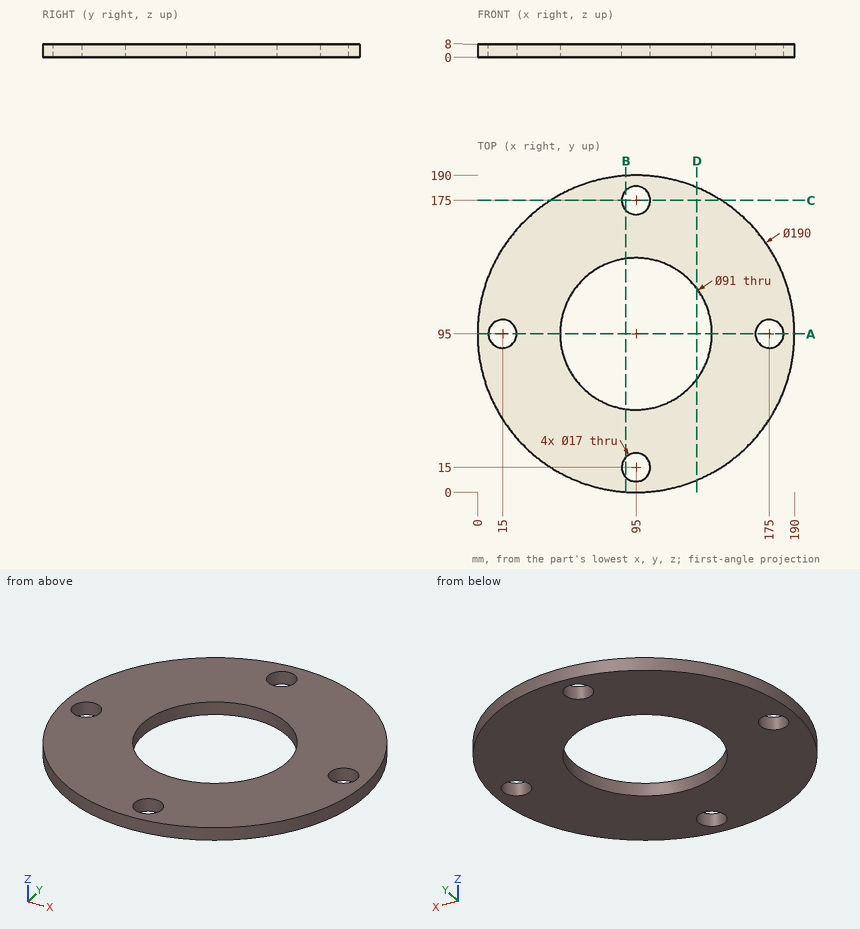
The figure shows three views and two pictorial views of one solid part (mm, origin at its lowest corner). Answer the questions. Give positions to 0.01 mm unless a question says otherwise; leave off trailing zeros. Write each loop counter-clockwise with the first axis right and the second up, starting at its lowest first coordinate (ties: lowest second). Pieces come first, ordered by that corner, then holes.
Q1. Given pin 1 (1 mm diameter, centred on y = 144.5, z = 5.5, fed in from +X); pin 2 (3 mm diameter, centred on x = 62.5, z = 5.5, fed in from +Y); pin 3 (15.5 mm diameter, centred on x = 15, y = 95, fed in from +Z); pin 4 (1.5 mm diameter, centred on x = 127, z = 3, fed in from +Y), each flat-ended and moving along its own axis, determine where each tip first touches the part or whether it passes through.
Answer:
pin 1: stops at x = 176.39
pin 2: stops at y = 184.8
pin 3: passes through
pin 4: stops at y = 184.71
Q2. The part is cut by section A-A on y = 95. Give the vertices of the cut face in (x, z).
Answer:
outline: (0, 0) - (6.5, 0) - (6.5, 8) - (0, 8) - close; (23.5, 0) - (49.5, 0) - (49.5, 8) - (23.5, 8) - close; (140.5, 0) - (166.5, 0) - (166.5, 8) - (140.5, 8) - close; (183.5, 0) - (190, 0) - (190, 8) - (183.5, 8) - close
Q3. The part is cut by section B-B on x = 89. Give the vertices of the cut face in (y, z), and give its area (3 significant figures).
Answer:
outline: (0.19, 0) - (8.98, 0) - (8.98, 8) - (0.19, 8) - close; (21.02, 0) - (49.9, 0) - (49.9, 8) - (21.02, 8) - close; (140.1, 0) - (168.98, 0) - (168.98, 8) - (140.1, 8) - close; (181.02, 0) - (189.81, 0) - (189.81, 8) - (181.02, 8) - close
area: 603 mm2
Q4. Straight lines are drawn through the part: L1, parallel to Y at x = 95.5, z = 7.5; L2, parallel to X at y = 17, z = 3; L3, parallel to Y at x = 73.5, z = 6.25. For each, find the intervals that lie inside material, in ascending order.
Answer:
L1: y = 0 to 6.51, 23.49 to 49.5, 140.5 to 166.51, 183.49 to 190
L2: x = 40.77 to 86.74, 103.26 to 149.23
L3: y = 2.46 to 54.9, 135.1 to 187.54
Q5. The part is cut by section C-C on y = 175. Give the vertices of the cut face in (x, z), and give its area (3 significant figures).
Answer:
outline: (43.77, 0) - (86.5, 0) - (86.5, 8) - (43.77, 8) - close; (103.5, 0) - (146.23, 0) - (146.23, 8) - (103.5, 8) - close
area: 684 mm2
Q6. The part is cut by section D-D on x = 131.5. Give the vertices of the cut face in (y, z).
Answer:
outline: (7.29, 0) - (67.83, 0) - (67.83, 8) - (7.29, 8) - close; (122.17, 0) - (182.71, 0) - (182.71, 8) - (122.17, 8) - close
